Geometry check sheet. Reference: drawing and pictorial views, mm from the part's lowest x, y, z. Give positions to 0.01 mm unless a question says otherwise; leave off trailing zeros. Write each loop counter-clockwise with the first axis right and the second up, starting at its lowest first coordinate (ties: lowest second). Pieces come first, ordered by that corner, then holes. Notation, with made-up numbers: M -36,-23 L 1,-23 A16 cw 1,4 Z; hole C 57.25,-20 d4. An arc over 180 degrees is marked long. Write item = value, one per line. Start each with the question number.
1) Cross-section at C-C, the plane y = 4.5. Record the cut outline in (x, z) (1 decimal), plus the area to 3 significant figures.
2) Scan lines: line 1 along Z through (x, y) = (12.7, 3); line 2 along X through (y, z) = (4.25, 4.5) (1 decimal); line 3 along X through (y, z) = (4.5, 6.75) (1 decimal). Record each from-to range of solid material in increasing order. Write a range as [from, to].
3) Cross-section at A-A, the plane x = 12.7. Record the cut outline in (y, z).
4) Go/stop test with flat-tipped pins: pin 1 (3 mm diameter, centred on y = 4, z = 3.5, fed in from -X); pin 2 (1.5 mm diameter, centred on y = 3, z = 5.5, fed in from -X). Record where each tip stops, or that it passes through.
5) Mould release check, pull along Z, two halves, no side actions. Record for the marked faces 1, 2 and 3: released by +Z, released by -Z, zero draft, split by the parting line, or undercut.
6) Cross-section at B-B, the plane z = 10.75. Record the cut outline in (x, y).
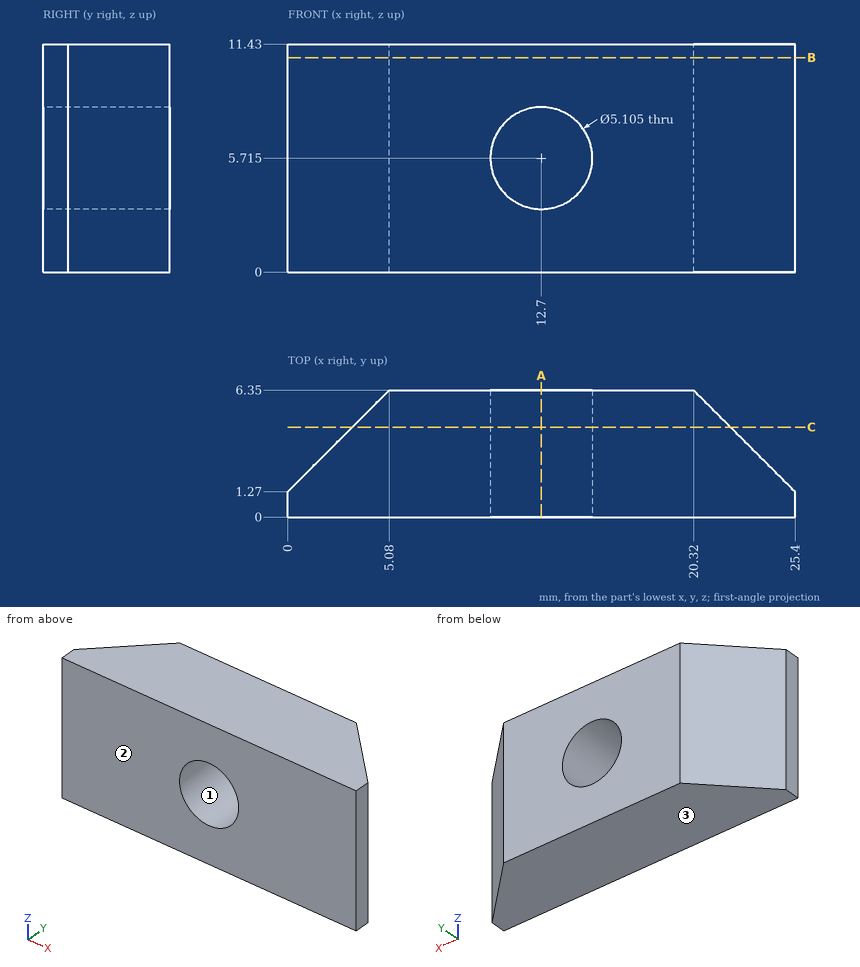
Reply:
q1.outline = M 3.2,0 L 22.2,0 L 22.2,11.4 L 3.2,11.4 Z; hole C 12.7,5.7 d5.1
q1.area = 196 mm2
q2.line_1 = [0, 3.16], [8.27, 11.43]
q2.line_2 = [3, 10.5], [14.9, 22.4]
q2.line_3 = [3.2, 10.4], [15, 22.2]
q3.outline = M 0,0 L 6.35,0 L 6.35,3.16 L 0,3.16 Z; M 0,8.27 L 6.35,8.27 L 6.35,11.43 L 0,11.43 Z
q4.pin_1 = 1.23
q4.pin_2 = 0.98
q5.face_1 = undercut
q5.face_2 = zero draft
q5.face_3 = released by -Z
q6.outline = M 0,0 L 25.4,0 L 25.4,1.27 L 20.32,6.35 L 5.08,6.35 L 0,1.27 Z
